```python
from build123d import *

# Parameters (mm, degrees)
SKETCH_1_W      = 33.4
SKETCH_1_H      = 8.02
EXTRUDE_1_DEPTH = 1
SKETCH_2_W      = 33.4
SKETCH_2_H      = 8.047596292
EXTRUDE_2_DEPTH = 1.5


with BuildPart() as part:
    # 스케치1 → 보스-돌출1 (new body)
    with BuildSketch(Plane.XY):
        Rectangle(SKETCH_1_W, SKETCH_1_H)
    extrude(amount=EXTRUDE_1_DEPTH)

    # 스케치2 → 보스-돌출2 (add)
    with BuildSketch(Plane.XY.offset(1)):
        Polygon((-16.7, 5.01), (17.743446376, 5.01), (17.743446376, 4.01), (17.743446376, -5.011), (16.7, -5.011), (-17.7, -5.011), (-17.7, -4.037596292), (-17.7, 5.01), align=None)
        with Locations((0, -0.013798146)):
            Rectangle(SKETCH_2_W, SKETCH_2_H, mode=Mode.SUBTRACT)
    extrude(amount=-EXTRUDE_2_DEPTH)


solid = part.part
```
Build history of the part. All positions in model axes, mm. A direction names the side the tool comes from. Give positions to 0.01 mm unless a question says otherwise; leave off trailing zeros. Order: outer loops, then holes, each group sorted by start corner. A loop starts at its lowest first (then second) coordinate and runs counter-clockwise, first axis right, second up. Notation, with made-up numbers: M 20,66.5 L 33,66.5 A18 cw 33,87.5 Z; hole C 27.25,53 d2. An arc over 180 degrees is marked long. Write item = value, one per line. Start each with the question number.
(1) Probe L1, parallel to Y at x = -7, z = -0.3; L2, parallel to X at y = 1.5, z = -0.25; L3, parallel to Z at x = -11, y = -1.25. List the from-to ranges inside material, lowest first. Write a range as [from, to].
(2) Slice it at A-A on x = -3. Write the cut outline in (y, z).
(3) Slice it at B-B on y = 2.5. Write the cut outline in (x, z).
(4) Two-plate mould, pull along X, no slides. Class faces 1 (the flat face through (17.743, 0, 0)), 2 (the flat face through (16.7, 0, -0.2)), 3 (the flat face through (0.1, -4.4, -0.5)): released by +X, released by -X, zero draft, split by the parting line, or undercut.
(5) Which spindle directions (+Z, -Z, +X, -X, +Y, -Y) get a long thin tool onto all of the face, cutting with end or side? Do faces 4 (the flat face through (0, 0, 0)), 5 (the flat face through (0, -5.011, 0)). Say none if no direction does.
(6) Pin check, flat tip, straight feed: pin 1 Ø6 at (x, y) = (9, -1) entering from -Z. Stop position of the tip, or through.
Responses:
q1.L1 = [-5.01, -4.04], [4.01, 5.01]
q1.L2 = [-17.7, -16.7], [16.7, 17.74]
q1.L3 = [0, 1]
q2.outline = M -5.01,-0.5 L -4.04,-0.5 L -4.04,1 L -5.01,1 Z; M -4.01,0 L 4.01,0 L 4.01,-0.5 L 5.01,-0.5 L 5.01,1 L -4.01,1 Z
q3.outline = M -17.7,-0.5 L -16.7,-0.5 L -16.7,0 L 16.7,0 L 16.7,-0.5 L 17.74,-0.5 L 17.74,1 L -17.7,1 Z
q4.face_1 = released by +X
q4.face_2 = undercut
q4.face_3 = zero draft
q5.face_4 = -Z
q5.face_5 = +Z, -Z, +X, -X, -Y
q6.pin_1 = 0
